Work out the finished part from the listing and answer in its coordinate system (mm). A direction names the side the tool comes from. Give positions to 0.01 mm unless a question says otherwise; leave off trailing zeros. Loops run counter-clockwise (first coordinate to the right, second up) from the corner with the lowest first, then second, coordinate; pieces in that order, holes last. Notation, with made-up numbers: M -10.5,52 L 0.5,52 A27 ccw 0.5,74 Z; hole C -7,78 d10. An arc over 180 degrees is marked long. Use a Markdown table: item, result.
```python
from build123d import *

# Parameters (mm, degrees)
SKETCH1_W           = 120.8
SKETCH1_H           = 50.8
BOSS_EXTRUDE1_DEPTH = 85.62
SKETCH2_W           = 24
SKETCH2_H           = 50.8
CUT_EXTRUDE1_DEPTH  = 60
SKETCH3_R           = 4
CUT_EXTRUDE2_DEPTH  = 121.8
SKETCH4_W           = 26.8
SKETCH4_H           = 60
CUT_EXTRUDE3_DEPTH  = 121.8


with BuildPart() as part:
    # Sketch1 → Boss-Extrude1 (new body)
    with BuildSketch(Plane.XY):
        with Locations((60.4, 25.4)):
            Rectangle(SKETCH1_W, SKETCH1_H)
    extrude(amount=BOSS_EXTRUDE1_DEPTH)

    # Sketch2 → Cut-Extrude1 (cut)
    with BuildSketch(Plane.XY.offset(85.62)):
        with Locations((60.4, 25.4)):
            Rectangle(SKETCH2_W, SKETCH2_H)
    extrude(amount=-CUT_EXTRUDE1_DEPTH, mode=Mode.SUBTRACT)

    # Sketch3 → Cut-Extrude2 (cut, through all)
    with BuildSketch(Plane.YZ.offset(120.8)):
        with Locations((38.8, 60.62)):
            Circle(SKETCH3_R)
    extrude(amount=-CUT_EXTRUDE2_DEPTH, mode=Mode.SUBTRACT)

    # Sketch4 → Cut-Extrude3 (cut, through all)
    with BuildSketch(Plane.YZ.offset(120.8)):
        with Locations((13.4, 55.62)):
            Rectangle(SKETCH4_W, SKETCH4_H)
    extrude(amount=-CUT_EXTRUDE3_DEPTH, mode=Mode.SUBTRACT)


solid = part.part
```
(1) Consider probe 1 along Z at (x, y) = (85, 38.8); probe 2 along X at (y, z) = (38, 49); probe 3 along Z at (x, y) = (100, 21). Determine where each line is inside the solid, lowest interval first. Write a range as [from, to].
Entries:
| item | result |
|---|---|
| probe 1 | z = [0, 56.62], [64.62, 85.62] |
| probe 2 | x = [0, 48.4], [72.4, 120.8] |
| probe 3 | z = [0, 25.62] |
(2) A cutting plane is placed at B-B (z = 40.5). Write down the section's boundary in (x, y).
Entries:
| item | result |
|---|---|
| outline | M 0,26.8 L 48.4,26.8 L 48.4,50.8 L 0,50.8 Z; M 72.4,26.8 L 120.8,26.8 L 120.8,50.8 L 72.4,50.8 Z |
(3) A cutting plane is placed at C-C (z = 60.62). Write down the section's boundary in (x, y), and give its area (3 significant figures).
Entries:
| item | result |
|---|---|
| outline | M 0,26.8 L 48.4,26.8 L 48.4,34.8 L 0,34.8 Z; M 0,42.8 L 48.4,42.8 L 48.4,50.8 L 0,50.8 Z; M 72.4,26.8 L 120.8,26.8 L 120.8,34.8 L 72.4,34.8 Z; M 72.4,42.8 L 120.8,42.8 L 120.8,50.8 L 72.4,50.8 Z |
| area | 1,550 mm² |
(4) A cutting plane is placed at A-A (y = 38.8). Write down the section's boundary in (x, z).
Entries:
| item | result |
|---|---|
| outline | M 0,0 L 120.8,0 L 120.8,56.62 L 72.4,56.62 L 72.4,25.62 L 48.4,25.62 L 48.4,56.62 L 0,56.62 Z; M 0,64.62 L 48.4,64.62 L 48.4,85.62 L 0,85.62 Z; M 72.4,64.62 L 120.8,64.62 L 120.8,85.62 L 72.4,85.62 Z |
(5) A cutting plane is placed at D-D (y = 33). Write down the section's boundary in (x, z), and give its area (3 significant figures).
Entries:
| item | result |
|---|---|
| outline | M 0,0 L 120.8,0 L 120.8,85.62 L 72.4,85.62 L 72.4,25.62 L 48.4,25.62 L 48.4,85.62 L 0,85.62 Z |
| area | 8,900 mm² |
(6) Which of the six approach directions +Z, -Z, +X, -X, +Y, -Y give full straight-line access (tool end or side, diameter ignored) to faces 5 (the flat face through (25, 26.8, 55)), 6 (the flat face through (72.4, 39, 56)), 7 (the flat face through (0, 31, 33))?
Entries:
| item | result |
|---|---|
| face 5 | +Z, +X, -X, -Y |
| face 6 | +Z, +Y, -Y |
| face 7 | +Z, -Z, -X, +Y, -Y |
(7) The mould has two halves that part along Z. Classify faces 1 (the flat face through (96, 39, 85.62)), 2 (the flat face through (60, 26, 0)), 3 (the flat face through (97, 26.8, 55)), 4 (the cylindrical face through (24.539, 40.95, 63.993)): released by +Z, released by -Z, zero draft, split by the parting line, or undercut.
Entries:
| item | result |
|---|---|
| face 1 | released by +Z |
| face 2 | released by -Z |
| face 3 | zero draft |
| face 4 | undercut |
(8) Given P1, Ø14.5, axis at x = 95.5, z = 55, coming from the -Y side; P2, Ø19, axis at y = 37, z = 63, coming from the -X side; P3, Ø5, axis at y = 38.8, z = 60.62, coming from the -X side; P4, Ø5, axis at x = 55, y = 33, coming from the +Z side, each flat-ended and moving along its own axis, determine where each tip first touches the part or whether it passes through.
Entries:
| item | result |
|---|---|
| P1 | stops at y = 26.8 |
| P2 | stops at x = 0 |
| P3 | passes through |
| P4 | stops at z = 25.62 |
